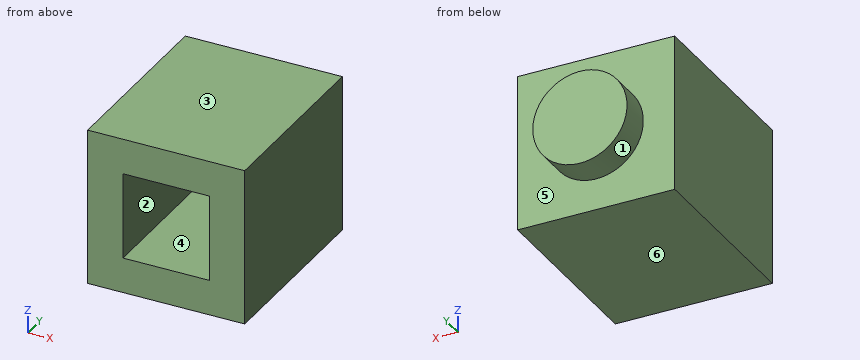
from build123d import *

# Parameters (mm, degrees)
SKETCH3_W           = 8
SKETCH3_H           = 8
BOSS_EXTRUDE1_DEPTH = 9.6
SKETCH4_R           = 2.4
BOSS_EXTRUDE2_DEPTH = 1.6
SHELL1_T            = -1.8


with BuildPart() as part:
    # Sketch3 → Boss-Extrude1 (new body)
    with BuildSketch(Plane(origin=(0, 0, 0), x_dir=(1, 0, 0), z_dir=(0, 1, 0))):
        with Locations((4, 4)):
            Rectangle(SKETCH3_W, SKETCH3_H)
    extrude(amount=BOSS_EXTRUDE1_DEPTH)

    # Sketch4 → Boss-Extrude2 (add)
    with BuildSketch(Plane(origin=(0, 9.6, 0), x_dir=(1, 0, 0), z_dir=(0, 1, 0))):
        with Locations((4, 4)):
            Circle(SKETCH4_R)
    extrude(amount=BOSS_EXTRUDE2_DEPTH)

    # Shell1
    shell1_openings = [part.faces().sort_by_distance(p)[0] for p in [
        (4, 0, -4),
    ]]
    offset(amount=SHELL1_T, openings=shell1_openings, kind=Kind.INTERSECTION)


solid = part.part
The model under review builds one solid part; all positions refer to its coordinate system, in mm. Face numbers are marked on the shaded views. A direction names the side the tool comes from. Round coordinates to 2 decimals unless told otherwise and drop trailing zeros. Loops run counter-clockwise (first coordinate to the right, second up) from the corner with the lowest first, then second, coordinate; pieces in that order, holes last. Notation, with made-up numbers: (-16.75, -33) - (-9.75, -33) arc R25 cw to (-9.75, -14) - close; hole circle Ø1 at (5, 61). An arc over 180 degrees is marked (long way). Use CSV: the item, a comma, the result in double quotes.
(1) The part is to be moulded in two halves that separate along X. For the marked faces 1, 2 and 3, say which applies: pulls with the +X half, pulls with the -X half, needs draft (parallel to the pull), parting line crosses it, or undercut.
Working result:
face 1,"parting line crosses it"
face 2,"undercut"
face 3,"needs draft"
(2) Take a section at A-A, the plane y = 5.5. Give the boundary of the cut face in (x, z).
Working result:
outline,"(0, -8) - (8, -8) - (8, 0) - (0, 0) - close; hole (1.8, -6.2) - (6.2, -6.2) - (6.2, -1.8) - (1.8, -1.8) - close"
(3) For line 1 (Z direction, x = 4, y = 8.7); line 2 (X direction, y = 1, z = -3); line 3 (Z direction, x = 2.75, y = 6.5), list the stretches that pass through material, from the lowest coordinate up.
Working result:
line 1,"z = -8 to -4.6, -3.4 to 0"
line 2,"x = 0 to 1.8, 6.2 to 8"
line 3,"z = -8 to -6.2, -1.8 to 0"
(4) Take a section at B-B, the plane z = -4. Give the boundary of the cut face in (x, y).
Working result:
outline,"(0, 0) - (1.8, 0) - (1.8, 7.8) - (3.4, 7.8) - (3.4, 9.4) - (4.6, 9.4) - (4.6, 7.8) - (6.2, 7.8) - (6.2, 0) - (8, 0) - (8, 9.6) - (6.4, 9.6) - (6.4, 11.2) - (1.6, 11.2) - (1.6, 9.6) - (0, 9.6) - close"
(5) Machinability: for the marked faces 4, 5 and 6, which of the approach directions +Z, -Z, +X, -X, +Y, -Y give a long, thin tool a straight path to every point of the face, cutting with its end or side? Answer none if there is none.
Working result:
face 4,"-Y"
face 5,"+Y"
face 6,"-Z, +X, -X, +Y, -Y"
(6) Take a section at C-C, the plane x = 4. Give the boundary of the cut face in (y, z).
Working result:
outline,"(0, -8) - (9.6, -8) - (9.6, -6.4) - (11.2, -6.4) - (11.2, -1.6) - (9.6, -1.6) - (9.6, 0) - (0, 0) - (0, -1.8) - (7.8, -1.8) - (7.8, -3.4) - (9.4, -3.4) - (9.4, -4.6) - (7.8, -4.6) - (7.8, -6.2) - (0, -6.2) - close"
(7) Clearance check with a flat-ended pin moving along its axis: P1, Ø1.3, axis at x = 3.5, z = -4.5, coming from the -Y side. State where the tip first meets the part, or that it passes through.
Working result:
P1,"stops at y = 7.8"
(8) Take a section at D-D, the plane x = 2. Give the boundary of the cut face in (y, z).
Working result:
outline,"(0, -8) - (9.6, -8) - (9.6, -5.33) - (11.2, -5.33) - (11.2, -2.67) - (9.6, -2.67) - (9.6, 0) - (0, 0) - (0, -1.8) - (7.8, -1.8) - (7.8, -6.2) - (0, -6.2) - close"
